Part model, mm, in its own coordinate system. Give positions to 0.01 mm unless a question says otherwise; leave off trailing zeros. Write item = value, one per line.
from build123d import *

# Parameters (mm, degrees)
SKETCH1_W           = 65.4
SKETCH1_H           = 3
BOSS_EXTRUDE1_DEPTH = 4
BOSS_EXTRUDE1_TAPER = 5
SKETCH2_R           = 1.2
CUT_EXTRUDE1_DEPTH  = 5.0000001
SKETCH3_R           = 2
CUT_EXTRUDE2_DEPTH  = 2


with BuildPart() as part:
    # Sketch1 → Boss-Extrude1 (new body)
    with BuildSketch(Plane.XY.offset(11.6)):
        with BuildLine():
            Line((-42.1, -10.1), (42.1, -10.1))
            ThreePointArc((42.1, -10.1), (42.807106781, -9.807106781), (43.1, -9.1))
            Line((43.1, -9.1), (43.1, 28.6))
            ThreePointArc((43.1, 28.6), (42.807106781, 29.307106781), (42.1, 29.6))
            Line((42.1, 29.6), (-42.1, 29.6))
            ThreePointArc((-42.1, 29.6), (-42.807106781, 29.307106781), (-43.1, 28.6))
            Line((-43.1, 28.6), (-43.1, -9.1))
            ThreePointArc((-43.1, -9.1), (-42.807106781, -9.807106781), (-42.1, -10.1))
        make_face()
        Rectangle(SKETCH1_W, SKETCH1_H, mode=Mode.SUBTRACT)
        with Locations((0, 19.5)):
            Rectangle(SKETCH1_W, SKETCH1_H, mode=Mode.SUBTRACT)
    extrude(amount=BOSS_EXTRUDE1_DEPTH, taper=BOSS_EXTRUDE1_TAPER)

    # Sketch2 → Cut-Extrude1 (cut, through all)
    with BuildSketch(Plane.XY.offset(15.6)):
        with Locations((-39.7, 26.2)):
            Circle(SKETCH2_R)
        with Locations((-39.7, -6.7)):
            Circle(SKETCH2_R)
        with Locations((39.7, -6.7)):
            Circle(SKETCH2_R)
        with Locations((39.7, 26.2)):
            Circle(SKETCH2_R)
    extrude(amount=-CUT_EXTRUDE1_DEPTH, mode=Mode.SUBTRACT)

    # Sketch3 → Cut-Extrude2 (cut)
    with BuildSketch(Plane.XY.offset(15.6)):
        with Locations((-39.7, 26.2)):
            Circle(SKETCH3_R)
        with Locations((-39.7, -6.7)):
            Circle(SKETCH3_R)
        with Locations((39.7, -6.7)):
            Circle(SKETCH3_R)
        with Locations((39.7, 26.2)):
            Circle(SKETCH3_R)
    extrude(amount=-CUT_EXTRUDE2_DEPTH, mode=Mode.SUBTRACT)


solid = part.part
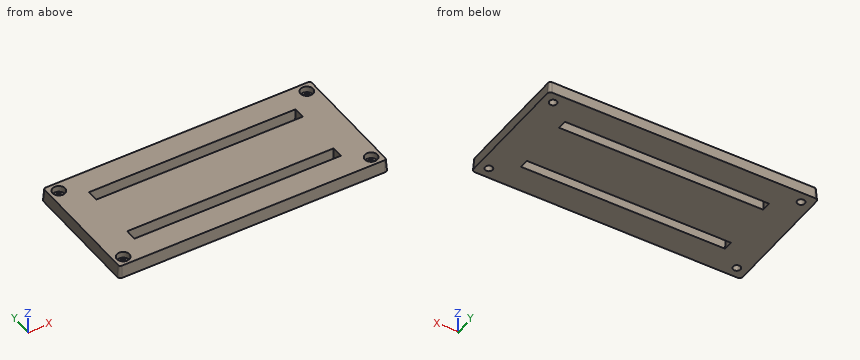
1) Slice it at A-A, the plane x = -28.5. Count the separate pieces of the cut face and the enclosed holes in it, and give its area (3 significant figures).
Resolved:
separate_pieces = 3
enclosed_holes = 0
area = 131 mm²
2) Drop flat-ended pins along their axis: P1, Ø3.5, axis at x = -39.7, y = -6.7, coming from the +Z side; P2, Ø1.5, axis at x = -27.5, z = 13, coming from the +Y side; P3, Ø1.5, axis at y = 17.5, z = 14, coming from the -X side. Give the stop position or say it passes through.
Resolved:
P1 = 13.6
P2 = 29.54
P3 = -42.96
3) Drill centre lines: line 1 along Y through (x, z) = (-3.5, 11.8); line 2 along Y through (x, z) = (17.5, 14.95); line 3 along X through (y, z) = (27.5, 14.6). Where is each one in solid material? Low to high. Write a range as [from, to].
Resolved:
line_1 = [-10.08, -1.52], [1.52, 17.98], [21.02, 29.58]
line_2 = [-9.81, -1.79], [1.79, 17.71], [21.29, 29.31]
line_3 = [-42.84, -41.22], [-38.18, 38.18], [41.22, 42.84]
